from build123d import *

# Parameters (mm, degrees)
F0_W     = 304.8
F0_H     = 203.2
F1_DEPTH = 19.05
F2_SIZE  = 50.8
F3_W     = 228.6
F3_H     = 25.4
F4_DEPTH = 19.05
F5_R     = 6.35
F7_D     = 6.35
F8_D     = 12.7
F8_DEPTH = 12.7
F8_TIP   = 3.8154649308
F9_D     = 9.525
F10_D    = 12.7


with BuildPart() as f1:
    # F0 (on Front) → F1 (new body)
    with BuildSketch(Plane.XZ):
        with Locations((22.3837513477, 30.5710117506)):
            Rectangle(F0_W, F0_H)
    extrude(amount=F1_DEPTH)

    # F2
    f2_edges = [f1.edges().sort_by_distance(p)[0] for p in [
        (-130.016249, -9.525, 132.171012),
        (174.783751, -9.525, 132.171012),
    ]]
    chamfer(f2_edges, length=F2_SIZE)

    # F3 (on face) → F4 (cut)
    with BuildSketch(Plane.XZ.offset(19.05)):
        with Locations((22.3837513477, -58.3289882494)):
            Rectangle(F3_W, F3_H)
    extrude(amount=-F4_DEPTH, mode=Mode.SUBTRACT)

    # F5
    f5_edges = [f1.edges().sort_by_distance(p)[0] for p in [
        (-130.016249, -9.525, -71.028988),
        (-91.916249, -9.525, -71.028988),
        (-91.916249, -9.525, -45.628988),
        (136.683751, -9.525, -71.028988),
        (174.783751, -9.525, -71.028988),
        (136.683751, -9.525, -45.628988),
    ]]
    fillet(f5_edges, radius=F5_R)

    # F7 (through all)
    with Locations(Plane.XZ.offset(19.05)):
        with Locations((98.5837513477, -32.9289882494), (35.0837513477, -32.9289882494)):
            Hole(F7_D / 2)

    # F8
    with Locations(Plane.XZ.offset(19.05)):
        with Locations((-104.6162486523, 63.1592117506), (149.3837513477, 63.1592117506), (-110.9662486523, 24.2210117506), (155.7337513477, 24.2210117506), (155.7337513477, -51.9789882494), (-110.9662486523, -51.9789882494)):
            Hole(F8_D / 2, depth=F8_DEPTH)
            with Locations((0, 0, -(F8_DEPTH + F8_TIP / 2))):  # 118° drill point
                Cone(0, F8_D / 2, F8_TIP, mode=Mode.SUBTRACT)

    # F9 (through all)
    with Locations(Plane.XZ.offset(19.05)):
        with Locations((-110.9662486523, 24.2210117506), (155.7337513477, 24.2210117506), (155.7337513477, -51.9789882494), (-110.9662486523, -51.9789882494)):
            Hole(F9_D / 2)

    # F10 (through all)
    with Locations(Plane.XZ.offset(19.05)):
        with Locations((22.3837513477, 33.8222117506)):
            Hole(F10_D / 2)


solid = f1.part
Input: part model. Units: mm. Frame: model coordinates. A direction names the side the tool comes from. Give positions to 0.01 mm unless a question says otherwise; leave off trailing zeros. Order: outer loops, then holes, each group sorted by start corner. A loop starts at its lowest first (then second) coordinate and runs counter-clockwise, first axis right, second up. Notation, with made-up numbers: (42, -31) - (77, -31) arc R15 cw to (77, -23) - close; hole circle Ø7 at (77, 30). An arc over 180 degrees is marked (long way). Answer as a JSON object with one key per item and string values. Group by question number.
Q1. Cut plane A-A, the plane x = -46.5. Output: boundary loops of the cut face in (y, z), then the cut area to 3 significant figures.
Q2. Mould query, pull axis Z, two halves, no side actions, for faces 1 (the face through (136.684, -10, -58)), 2 (the face through (148.28, -3.2, 63.21)), 3 (the face through (149.028, -9.392, 107.127)). Classes: pulls with the +Z half, pulls with the -Z half, needs draft (parallel to the pull), parting line crosses it, or undercut.
Q3. Set-up query: faces 4 (the face through (-103.24, -12.61, 56.96)), 5 (the face through (138.593, -9.392, -69.218)), 6 (the face through (160.49, -2.66, -51.77)). Return all of +Z, -Z, +X, -X, +Y, -Y with unobstructed straight access to the full face (end or side cutting, diameter ignored); none if empty.
Q4. First-contact query: pin 1 Ø5 at (x, y) = (-36.5, -10.5) entering from -Z; pin 2 Ø8 at (y, z) = (-11, 107.5) entering from -X. Flat tips, straight axial feed; report the tip coordinate or a pass-through.
Q5. Line query: probe 1 along X at (y, z) = (-15.75, 23); probe 2 along X at (y, z) = (-15.25, 66); probe 3 along Z at (x, y) = (-76.5, -2). Output: solid intervals per line, ascending.
Q6. Cut plane B-B, the plane z = 118.5. Output: boundary loops of the cut face in (x, y).
Results:
{
 "1": {"outline": "(-19.05, -45.63) - (0, -45.63) - (0, 132.17) - (-19.05, 132.17) - close", "area": "3,390 mm^2"},
 "2": {"face 1": "needs draft", "face 2": "undercut", "face 3": "pulls with the +Z half"},
 "3": {"face 4": "-Y", "face 5": "-Z, +Y, -Y", "face 6": "+Y, -Y"},
 "4": {"pin 1": "z = -45.63", "pin 2": "x = -107.89"},
 "5": {"probe 1": "-130.02 to -117.2, -104.73 to 149.5, 161.97 to 174.78", "probe 2": "-130.02 to -110.3, -98.94 to 143.7, 155.06 to 174.78", "probe 3": "-45.63 to 132.17"},
 "6": {"outline": "(-92.89, -19.05) - (137.65, -19.05) - (137.65, 0) - (-92.89, 0) - close"}
}
